The drawing under review shows one solid part. Ordinate dimensions are in mm from its lowest x, y, z. A direction names the side the tool comes from. Give positions to 0.01 mm unless a question says otherwise; leave off trailing zeros. Loops run counter-clockwise (first coordinate to the right, second up) from the corner with the lowest first, then second, coordinate; pieces in that order, holes last.
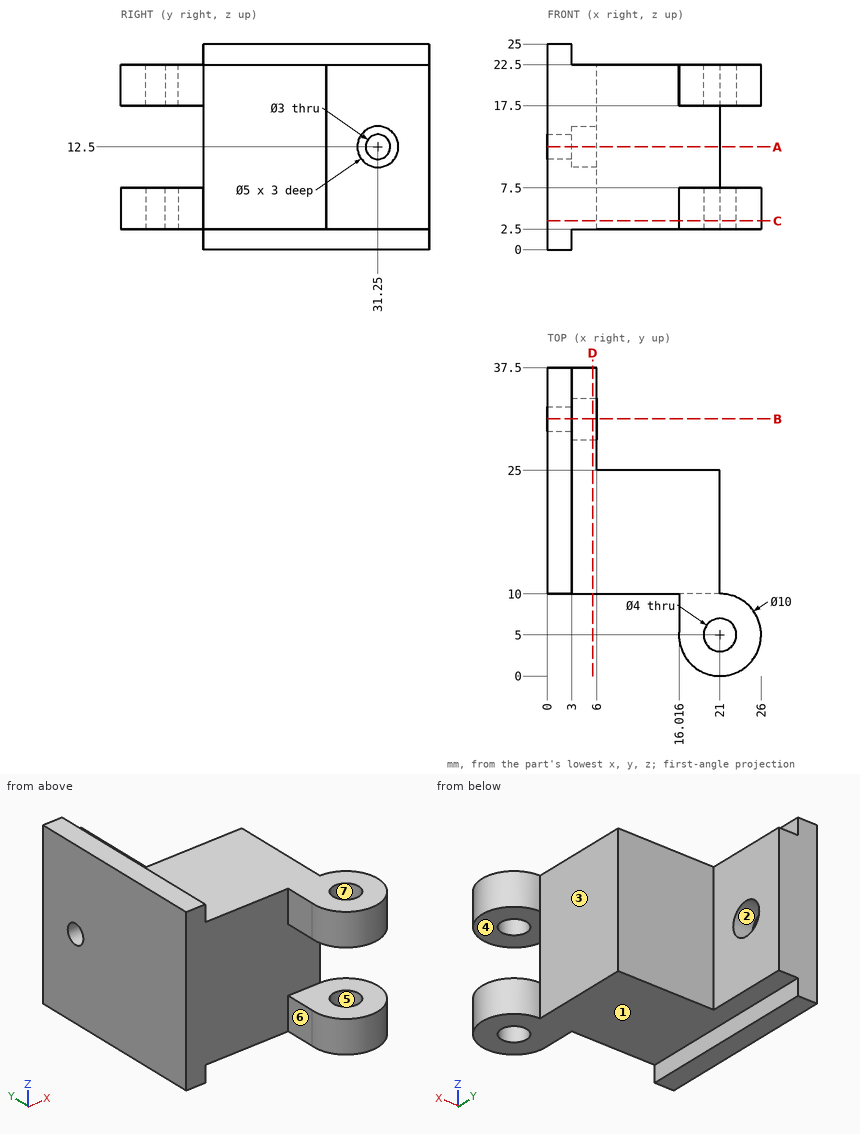
Item 1: Clearance check with flat-ended pins moving along their axes: pin 1 Ø8 at (x, z) = (16, 15.5) entering from -Y; pin 2 Ø1 at (x, z) = (7.5, 14) entering from +Y; pin 3 Ø0.8 at (y, z) = (28, 24) entering from +X; pin 4 Ø6.5 at (y, z) = (31.25, 12.5) entering from -X. State where each tip first meets the part, or that it passes through.
Answer:
pin 1: stops at y = 0.24
pin 2: stops at y = 25
pin 3: stops at x = 3
pin 4: stops at x = 0
Item 2: Take a section at B-B on y = 31.25. Give the boundary of the cut face in (x, z), and give its area (3 significant figures).
Answer:
outline: (0, 0) - (3, 0) - (3, 2.5) - (6, 2.5) - (6, 10) - (3, 10) - (3, 11) - (0, 11) - close; (0, 14) - (3, 14) - (3, 15) - (6, 15) - (6, 22.5) - (3, 22.5) - (3, 25) - (0, 25) - close
area: 111 mm2
Item 3: The part is to be moulded in two halves that separate along X. For the marked faces 4, 5, 6 and 7, say which applies: released by +X, released by -X, zero draft, split by the parting line, or undercut.
Answer:
face 4: zero draft
face 5: undercut
face 6: released by -X
face 7: undercut
Item 4: Take a section at D-D on x = 5.5. Give the boundary of the cut face in (y, z).
Answer:
outline: (10, 2.5) - (37.5, 2.5) - (37.5, 22.5) - (10, 22.5) - close; hole circle Ø5 at (31.25, 12.5)
Item 5: Take a section at C-C on z = 3.5. Give the boundary of the cut face in (x, y) (1 decimal).
Answer:
outline: (0, 10) - (16, 10) - (16, 5.4) arc R5 ccw (long way) to (21, 10) - (21, 25) - (6, 25) - (6, 37.5) - (0, 37.5) - close; hole circle Ø4 at (21, 5)
Item 6: Tool access review of the marked faces 1, 2 and 3: name each direction out of +Z, -Z, +X, -X, +Y, -Y from which nothing blocks a thin tool from reaching the whole face with its end or side.
Answer:
face 1: -Z, +X, +Y, -Y
face 2: +X
face 3: +Z, -Z, +X, +Y
Item 7: For L1, parallel to Z at x = 4.05, y = 31.25; L2, parallel to Y at x = 3.7, z = 12.5; L3, parallel to Z at x = 24, y = 2.5, list the stretches that pass through material, from the lowest coordinate up.
Answer:
L1: z = 2.5 to 10, 15 to 22.5
L2: y = 10 to 28.75, 33.75 to 37.5
L3: z = 2.5 to 7.5, 17.5 to 22.5
Item 8: Take a section at A-A on z = 12.5. Give the boundary of the cut face in (x, y), and give its area (3 significant figures).
Answer:
outline: (0, 10) - (21, 10) - (21, 25) - (6, 25) - (6, 28.75) - (3, 28.75) - (3, 29.75) - (0, 29.75) - close; (0, 32.75) - (3, 32.75) - (3, 33.75) - (6, 33.75) - (6, 37.5) - (0, 37.5) - close
area: 366 mm2
